Can you work these out from the drawing? Everything is in mm from the part's minimum corner. Round coordinates to 2 decimals unless told otherwise and drop trailing zeros. Loops run counter-clockwise (first coordinate to the right, second up) from the corner with the lowest first, then second, coordinate; pieces in that order, holes last. Notation, with made-up numbers: M -33,11.5 L 16,11.5 A22 ccw 16,19.5 Z; hole C 28,84.25 d2. An arc over 180 degrees is marked long. Answer in a Markdown table with one row per item.
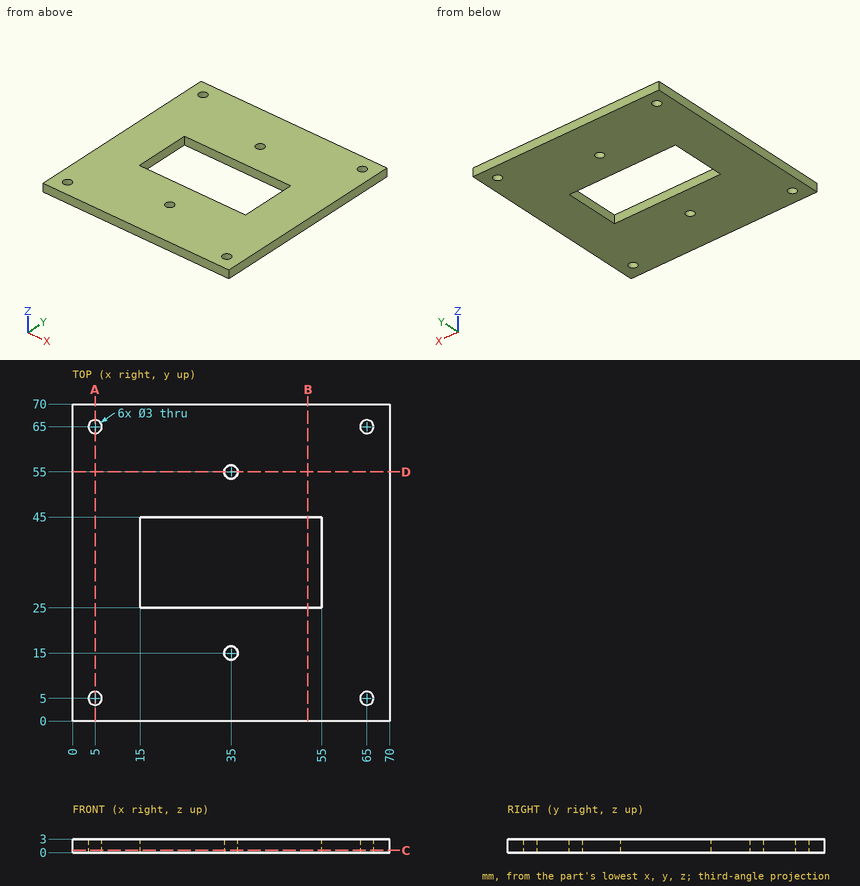
1) I want a section at A-A, the plane x = 5. Please give me the cut outline in (y, z), plus the area to 3 significant figures.
Computed:
| item | result |
|---|---|
| outline | M 0,0 L 3.5,0 L 3.5,3 L 0,3 Z; M 6.5,0 L 63.5,0 L 63.5,3 L 6.5,3 Z; M 66.5,0 L 70,0 L 70,3 L 66.5,3 Z |
| area | 192 mm² |
2) Will this pin go through, and if not, where does the flat tip stop? P1, Ø1.8, axis at x = 65, y = 5, coming from the -Z side.
Computed:
| item | result |
|---|---|
| P1 | passes through |
3) I want a section at C-C, the plane z = 0.5. Please give me the cut outline in (x, y).
Computed:
| item | result |
|---|---|
| outline | M 0,0 L 70,0 L 70,70 L 0,70 Z; hole C 5,5 d3; hole C 5,65 d3; hole M 15,25 L 55,25 L 55,45 L 15,45 Z; hole C 35,15 d3; hole C 35,55 d3; hole C 65,5 d3; hole C 65,65 d3 |
4) I want a section at D-D, the plane y = 55. Please give me the cut outline in (x, z), plus the area to 3 significant figures.
Computed:
| item | result |
|---|---|
| outline | M 0,0 L 33.5,0 L 33.5,3 L 0,3 Z; M 36.5,0 L 70,0 L 70,3 L 36.5,3 Z |
| area | 201 mm² |
5) I need wall thicknesses on line 1 (X direction, y = 65, z = 0.85); line 2 (Y direction, x = 35, z = 2.3); line 3 (X direction, y = 27.5, z = 0.9). Which ranges of each line are inside material? Lowest first, please.
Computed:
| item | result |
|---|---|
| line 1 | x = 0 to 3.5, 6.5 to 63.5, 66.5 to 70 |
| line 2 | y = 0 to 13.5, 16.5 to 25, 45 to 53.5, 56.5 to 70 |
| line 3 | x = 0 to 15, 55 to 70 |
6) I want a section at B-B, the plane x = 52. Please give me the cut outline in (y, z).
Computed:
| item | result |
|---|---|
| outline | M 0,0 L 25,0 L 25,3 L 0,3 Z; M 45,0 L 70,0 L 70,3 L 45,3 Z |
